Verification items for this drawing (mm, ordinates from the low corner). Coordinates: 2 decimals unless noted, no trailing zeros. Loops run counter-clockwise (first coordinate to the right, second up) from the corner with the lowest first, then second, coordinate; pieces in that order, holes last. Notation, with made-up numbers: M 8.5,18 L 57.5,18 A8 ccw 57.5,29 Z; hole C 54.25,14.5 d3. An arc over 180 degrees is marked long. Return JSON: item names as keys, results as strings.
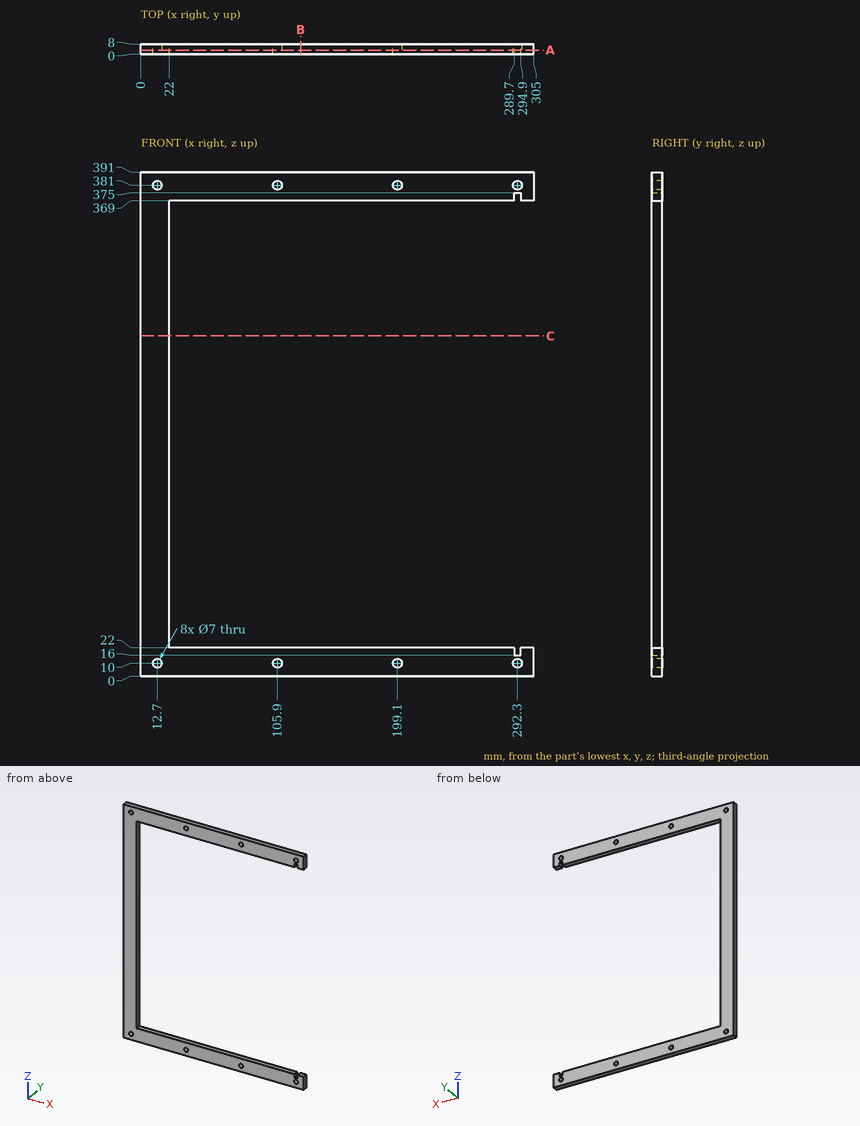
1) Section check B-B on x = 124. Record the cut outline in (y, z).
Answers:
{"outline": "M 0,0 L 8,0 L 8,22 L 0,22 Z; M 0,369 L 8,369 L 8,391 L 0,391 Z"}
2) Scan lines: line 1 along Z through (x, y) = (292, 0.5); line 2 along X through (y, z) = (5, 381); line 3 along Z through (x, y) = (105.9, 1.5). Record each from-to range of solid material in increasing order. Write a range as [from, to].
Answers:
{"line 1": "[0, 6.51], [13.49, 16], [375, 377.51], [384.49, 391]", "line 2": "[0, 9.2], [16.2, 102.4], [109.4, 195.6], [202.6, 288.8], [295.8, 305]", "line 3": "[0, 6.5], [13.5, 22], [369, 377.5], [384.5, 391]"}
3) Go/stop test with flat-tipped pins: pin 1 Ø2 at (y, z) = (1, 287.5) entering from +X; pin 2 Ø4 at (x, z) = (105.9, 10) entering from -Y. Record where each tip stops, or that it passes through.
Answers:
{"pin 1": "x = 22", "pin 2": "through"}
4) Section check A-A on y = 3.25. Count the separate pieces of the cut face and the enclosed holes in it, then the cut area to 3 significant figures.
Answers:
{"separate pieces": "1", "enclosed holes": "8", "area": "20,700 mm²"}
5) Section check C-C on z = 264. Record the cut outline in (x, y), then the cut area to 3 significant figures.
Answers:
{"outline": "M 0,0 L 22,0 L 22,8 L 0,8 Z", "area": "176 mm²"}
